```python
from build123d import *

# Parameters (mm, degrees)
SKETCH1_W           = 16.637
SKETCH1_H           = 16.637
BOSS_EXTRUDE1_DEPTH = 28.067
SKETCH2_W           = 19.304
SKETCH2_H           = 19.304
BOSS_EXTRUDE2_DEPTH = 19.304
SKETCH3_W           = 16.637
SKETCH3_H           = 16.637
BOSS_EXTRUDE3_DEPTH = 28.067
FILLET1_R           = 1.27


with BuildPart() as part:
    # Sketch1 → Boss-Extrude1 (new body)
    with BuildSketch(Plane(origin=(0, 0, 0), x_dir=(1, 0, 0), z_dir=(0, 1, 0))):
        Rectangle(SKETCH1_W, SKETCH1_H)
    extrude(amount=BOSS_EXTRUDE1_DEPTH)

    # Sketch2 → Boss-Extrude2 (add)
    with BuildSketch(Plane(origin=(0, 28.067, 0), x_dir=(1, 0, 0), z_dir=(0, 1, 0))):
        Rectangle(SKETCH2_W, SKETCH2_H)
    extrude(amount=BOSS_EXTRUDE2_DEPTH)

    # Sketch3 → Boss-Extrude3 (add)
    with BuildSketch(Plane.XY.offset(9.652)):
        with Locations((0, 37.719)):
            Rectangle(SKETCH3_W, SKETCH3_H)
    extrude(amount=BOSS_EXTRUDE3_DEPTH)

    # Fillet1
    fillet1_edges = [part.edges().sort_by_distance(p)[0] for p in [
        (9.652, 37.719, -9.652),
        (-9.652, 37.719, -9.652),
        (9.652, 47.371, 0),
        (0, 47.371, -9.652),
        (-9.652, 47.371, 0),
        (8.3185, 29.4005, 23.6855),
        (8.3185, 46.0375, 23.6855),
        (-8.3185, 46.0375, 23.6855),
        (-8.3185, 29.4005, 23.6855),
        (8.3185, 14.0335, 8.3185),
        (-8.3185, 14.0335, 8.3185),
        (-8.3185, 14.0335, -8.3185),
        (8.3185, 14.0335, -8.3185),
    ]]
    fillet(fillet1_edges, radius=FILLET1_R)


solid = part.part
```
The model under review builds one solid part; all positions refer to its coordinate system, in mm. A direction names the side the tool comes from. Round coordinates to 2 decimals unless told otherwise and drop trailing zeros. Write each loop counter-clockwise with the first axis right and the second up, starting at its lowest first coordinate (ties: lowest second). Pieces come first, ordered by that corner, then holes. Notation, with made-up numbers: (3, -28.75) - (22, -28.75) arc R14 ccw to (22, -6.75) - close; hole circle Ø3 at (-6.5, 37.25). An arc over 180 degrees is marked (long way). Answer as CSV lines item,"result". Start each with the question number.
(1) To check wall thickness, follow line 1 (Z direction, x = -2, y = 20); line 2 (Y direction, x = 5, z = 35.5). State the ranges of each line that lie inside material, in increasing order.
(2) For faces 1 (the flat face through (0, 14, 8.318)), 2 (the flat face through (8.318, 38, 23)), 3 (the cylindrical face through (7.956, 14.23, -7.937)), 4 (the cylindrical face through (7.937, 45.675, 23.882)), 5 (the flat face through (-0.1, 46.2, 9.652)), list the 3-axis set-ups (+Z, -Z, +X, -X, +Y, -Y) from which the entire face can be reached by the end or side of a thin tool; tool diameter is ignored.
(3) We need section D-D on z = 2. State the section outline as (x, y) points.
(4) We need section B-B on y = 14.5. State the section outline as (x, z) points, plus the area to 3 significant figures.
(5) We need section A-A on z = 35.5. State the section outline as (x, y) points.
(6) For pin 1 Ø7 at (y, z) = (11, -3) entering from +X; pin 2 Ø10 at (x, z) = (-6.5, 17) entering from +Y; pin 3 Ø3 at (y, z) = (42, 21.5) entering from -X, all flat-tipped, find the tip position at first contact; note any pin that passes through.
(7) We need section C-C on x = -5. State the section outline as (y, z) points.
Worked answers:
1,line 1,"-8.32 to 8.32"
1,line 2,"29.4 to 46.04"
2,face 1,"+Z, +X, -X, -Y"
2,face 2,"+Z, +X, +Y, -Y"
2,face 3,"-Z, +X, -Y"
2,face 4,"+Z, +X, +Y"
2,face 5,"+Z"
3,outline,"(-9.65, 28.07) - (-8.32, 28.07) - (-8.32, 0) - (8.32, 0) - (8.32, 28.07) - (9.65, 28.07) - (9.65, 46.1) arc R1.27 ccw to (8.38, 47.37) - (-8.38, 47.37) arc R1.27 ccw to (-9.65, 46.1) - close"
4,outline,"(-8.32, -7.05) arc R1.27 ccw to (-7.05, -8.32) - (7.05, -8.32) arc R1.27 ccw to (8.32, -7.05) - (8.32, 7.05) arc R1.27 ccw to (7.05, 8.32) - (-7.05, 8.32) arc R1.27 ccw to (-8.32, 7.05) - close"
4,area,"275 mm²"
5,outline,"(-8.32, 30.67) arc R1.27 ccw to (-7.05, 29.4) - (7.05, 29.4) arc R1.27 ccw to (8.32, 30.67) - (8.32, 44.77) arc R1.27 ccw to (7.05, 46.04) - (-7.05, 46.04) arc R1.27 ccw to (-8.32, 44.77) - close"
6,pin 1,"x = 8.32"
6,pin 2,"y = 46.04"
6,pin 3,"x = -8.32"
7,outline,"(0, -8.32) - (28.07, -8.32) - (28.07, -9.65) - (46.1, -9.65) arc R1.27 ccw to (47.37, -8.38) - (47.37, 9.65) - (46.04, 9.65) - (46.04, 37.72) - (29.4, 37.72) - (29.4, 9.65) - (28.07, 9.65) - (28.07, 8.32) - (0, 8.32) - close"
